For this review, take the finished solid that the model builds, in its own axes (mm). A direction names the side the tool comes from. Give positions to 0.01 mm unless a question says otherwise; leave off trailing zeros. Order: outer loops, then holes, each group sorted by start corner. A loop starts at its lowest first (then second) coordinate and runs counter-clockwise, first axis right, second up.
Item 1: Consider section C-C (x = 16.5). Give the boundary of the cut face in (y, z).
Item 2: Consider section D-D (y = 13). Give the boundary of the cut face in (x, z), plus the area to 3 significant figures.
Item 3: For probe 1 along Y at (x, z) = (22.26, 0.65); probe 2 along Y at (x, z) = (9.56, 1.3); probe 3 along Z at (x, y) = (37, 21.5), list the stretches that pass through material, from the lowest coordinate up.
Item 4: Consider section B-B (y = 3.81). Give the boundary of the cut face in (x, z).
Item 5: The part is to be moulded in two halves that separate along X. For faces 1 (the cylindrical face through (16.96, -21.61, -1.48)), 2 (the cylindrical face through (2.066, 0.35, 1.804)), 3 (the cylindrical face through (14.43, 12.61, 0.99)), 4 (the flat face through (18.926, -13, 1)), say which applies: released by +X, released by -X, zero draft, split by the parting line, or undercut.
Item 6: For P1, Ø5, axis at x = 17.18, y = 12.7, coming from the -Z side; P2, Ø1.5, axis at y = -3, z = 0.5, coming from the +X side; P3, Ø0.6, axis at y = 13.5, z = 1.5, coming from the -X side, all flat-tipped, find the tip position at first contact; note any pin that passes through.
Item 7: Machinability: for faces 5 (the cylindrical face through (16.96, 23.39, -1.48)), 6 (the cylindrical face through (25.31, 5.07, 0.99)), which of the approach directions +Z, -Z, +X, -X, +Y, -Y give a long, thin tool a straight path to every point of the face, cutting with its end or side? Answer none if there is none.
Item 8: Consider section A-A (x = 9.56). Give the boundary of the cut face in (y, z).
```python
from build123d import *

# Parameters (mm, degrees)
PAD_DEPTH     = 25
SKETCH001_R   = 1
PAD001_DEPTH  = 3
SKETCH002_R   = 2.55
SKETCH002_R_2 = 3.3
POCKET_DEPTH  = 2.001
FILLET_R      = 2.5


with BuildPart() as part:
    # Sketch → Pad (new body, symmetric)
    with BuildSketch(Plane.XZ):
        Polygon((0, 0), (2, 2), (38.599585, 2), (40, 0), align=None)
    extrude(amount=PAD_DEPTH, both=True)

    # Sketch001 (on Face4 of Pad) → Pad001 (join)
    with BuildSketch(Plane(origin=(0, 0, 0), x_dir=(1, 0, 0), z_dir=(0, 0, -1))):
        with Locations((16.5, 22.5)):
            Circle(SKETCH001_R)
        with Locations((16.5, -22.5)):
            Circle(SKETCH001_R)
    extrude(amount=PAD001_DEPTH)

    # Sketch002 (on Face2 of Pad001) → Pocket (cut, through all)
    with BuildSketch(Plane(origin=(0, 0, 0), x_dir=(1, 0, 0), z_dir=(0, 0, -1))):
        with Locations((9.56, 16.51)):
            Circle(SKETCH002_R)
        with Locations((9.56, 8.89)):
            Circle(SKETCH002_R)
        with Locations((9.56, -8.89)):
            Circle(SKETCH002_R)
        with Locations((9.56, -16.51)):
            Circle(SKETCH002_R)
        with Locations((22.26, 3.81)):
            Circle(SKETCH002_R_2)
        with Locations((22.26, -3.81)):
            Circle(SKETCH002_R_2)
        with BuildLine():
            Line((18.92553, 14.825), (18.92553, 10.575))
            ThreePointArc((18.92553, 14.825), (14.43, 12.7), (18.92553, 10.575))
        make_face()
        with BuildLine():
            Line((18.92553, -10.575), (18.92553, -14.825))
            ThreePointArc((18.92553, -10.575), (14.43, -12.7), (18.92553, -14.825))
        make_face()
    extrude(amount=-POCKET_DEPTH, mode=Mode.SUBTRACT)

    # Fillet
    fillet_edges = [part.edges().sort_by_distance(p)[0] for p in [
        (38.599585, 0, 2),
        (2, 0, 2),
    ]]
    fillet(fillet_edges, radius=FILLET_R)


solid = part.part
```
Resolved:
1. outline: (-25, 0) - (-23.5, 0) - (-23.5, -3) - (-21.5, -3) - (-21.5, 0) - (-15.36, 0) - (-15.36, 2) - (-25, 2) - close; (-10.04, 0) - (10.04, 0) - (10.04, 2) - (-10.04, 2) - close; (15.36, 0) - (21.5, 0) - (21.5, -3) - (23.5, -3) - (23.5, 0) - (25, 0) - (25, 2) - (15.36, 2) - close
2. outline: (0, 0) - (14.45, 0) - (14.45, 2) - (3.04, 2) arc R2.5 ccw to (1.27, 1.27) - close; (18.93, 0) - (40, 0) - (39.35, 0.93) arc R2.5 ccw to (37.3, 2) - (18.93, 2) - close
2. area: 67.3 mm2
3. probe 1: y = -25 to -7.11, -0.51 to 0.51, 7.11 to 25
3. probe 2: y = -25 to -19.06, -13.96 to -11.44, -6.34 to 6.34, 11.44 to 13.96, 19.06 to 25
3. probe 3: z = 0 to 2
4. outline: (0, 0) - (18.96, 0) - (18.96, 2) - (3.04, 2) arc R2.5 ccw to (1.27, 1.27) - close; (25.56, 0) - (40, 0) - (39.35, 0.93) arc R2.5 ccw to (37.3, 2) - (25.56, 2) - close
5. face 1: split by the parting line
5. face 2: released by -X
5. face 3: undercut
5. face 4: undercut
6. P1: stops at z = 0
6. P2: stops at x = 40
6. P3: stops at x = 1.2
7. face 5: -Z
7. face 6: +Z, -Z
8. outline: (-25, 0) - (-19.06, 0) - (-19.06, 2) - (-25, 2) - close; (-13.96, 0) - (-11.44, 0) - (-11.44, 2) - (-13.96, 2) - close; (-6.34, 0) - (6.34, 0) - (6.34, 2) - (-6.34, 2) - close; (11.44, 0) - (13.96, 0) - (13.96, 2) - (11.44, 2) - close; (19.06, 0) - (25, 0) - (25, 2) - (19.06, 2) - close
